Design review of the part built by this model. Coordinates are the model's own, in mm. A direction names the side the tool comes from. Coordinates: 2 decimals unless noted, no trailing zeros. Write each loop counter-clockwise with the first axis right and the second up, starting at its lowest first coordinate (ties: lowest second). Pieces come first, ordered by that corner, then holes.
Q1. Take a section at B-B (y = 12). Give the boundary of the cut face in (x, z), and give its area (3 significant figures).
Q2. Machinability: for faces 1 (the flat face through (0, 12, 12.5)), 2 (the flat face through (48, 0, 6)), 3 (the flat face through (-48, 0, -6)), which of the approach directions +Z, -Z, +X, -X, +Y, -Y give a long, thin tool a straight path to every point of the face, cutting with its end or side? Answer none if there is none.
Q3. For probe 1 along X at (y, z) = (-0.9, 0); probe 2 along Y at (x, z) = (0, 10); probe 3 along Z at (x, y) = (50, -1.3), list the stretches that pass through material, from the lowest coordinate up.
Q4. Mouldability with a two-part tool opening along X and no side actions: class faces 4 (the flat face through (-40, 0, 18)), 5 (the cylindrical face through (-45.043, -0.035, -0.651)), 6 (the flat face through (9.78, 11.13, 10.04)) as pulls with the +X half, pulls with the -X half, needs draft (parallel to the pull), parting line crosses it, or undercut.
Q5. Take a section at A-A (x = 0). Give the boundary of the cut face in (y, z), and give its area (3 significant figures).
Q6. Insertion check: pin 1 (4 mm diameter, centred on y = 0, z = 19, fed in from +X); pin 2 (4 mm diameter, centred on x = -47, y = 1, fed in from +Z); pin 3 (1.5 mm diameter, centred on x = 47, y = 1, fed in from -Z); pin 4 (8 mm diameter, centred on x = 50, z = 0, fed in from -Y). Each pin has a flat end and moves straight along its axis. Give the tip position at first contact, or say it passes through.
Q7. Take a section at D-D (z = -34). Give the boundary of the cut face in (x, y).
Q8. Take a section at C-C (y = 23.75). Give the boundary of the cut face in (x, z).
```python
from build123d import *

# Parameters (mm, degrees)
SKETCH1_R           = 5
BOSS_EXTRUDE1_DEPTH = 2.5
FILLET1_R           = 5
BOSS_EXTRUDE2_START = 10
BOSS_EXTRUDE2_DEPTH = 2.5
BOSS_EXTRUDE3_START = -10
BOSS_EXTRUDE3_DEPTH = 2.5
SKETCH3_R           = 5
CUT_EXTRUDE1_DEPTH  = 85


with BuildPart() as part:
    # Sketch1 → Boss-Extrude1 (new, symmetric)
    with BuildSketch(Plane(origin=(0, 0, 0), x_dir=(1, 0, 0), z_dir=(0, 1, 0))):
        with BuildLine():
            Line((-40, 6), (-56, 6))
            Line((-56, 6), (-56, -6))
            Line((-56, -6), (-40, -6))
            Line((-40, -6), (-40, -25))
            ThreePointArc((-40, -25), (-35.606601718, -35.606601718), (-25, -40))
            Line((-25, -40), (25, -40))
            ThreePointArc((25, -40), (35.606601718, -35.606601718), (40, -25))
            Line((40, -25), (40, -6))
            Line((40, -6), (56, -6))
            Line((56, -6), (56, 6))
            Line((56, 6), (40, 6))
            Line((40, 6), (40, 25))
            ThreePointArc((40, 25), (35.606601718, 35.606601718), (25, 40))
            Line((25, 40), (-25, 40))
            ThreePointArc((-25, 40), (-35.606601718, 35.606601718), (-40, 25))
            Line((-40, 25), (-40, 6))
        make_face()
        with Locations(Location((-50, 0, 0), (0, 0, 270))):
            Circle(SKETCH1_R, mode=Mode.SUBTRACT)
        with Locations(Location((50, 0, 0), (0, 0, 90))):
            Circle(SKETCH1_R, mode=Mode.SUBTRACT)
    extrude(amount=BOSS_EXTRUDE1_DEPTH, both=True)

    # Fillet1
    fillet1_edges = [part.edges().sort_by_distance(p)[0] for p in [
        (40, 0, -6),
        (56, 0, -6),
        (56, 0, 6),
        (40, 0, 6),
        (-40, 0, 6),
        (-56, 0, 6),
        (-56, 0, -6),
        (-40, 0, -6),
    ]]
    fillet(fillet1_edges, radius=FILLET1_R)

    # Sketch2 → Boss-Extrude2 (add, symmetric)
    with BuildSketch(Plane.XY.offset(BOSS_EXTRUDE2_START)):
        with BuildLine():
            Line((-7.5, 20), (-12, 2.5))
            Line((-12, 2.5), (12, 2.5))
            Line((12, 2.5), (7.5, 20))
            ThreePointArc((7.5, 20), (0, 27.5), (-7.5, 20))
        make_face()
    extrude(amount=BOSS_EXTRUDE2_DEPTH, both=True)

    # Sketch2_2 → Boss-Extrude3 (add, symmetric)
    with BuildSketch(Plane.XY.offset(BOSS_EXTRUDE3_START)):
        with BuildLine():
            Line((-7.5, 20), (-12, 2.5))
            Line((-12, 2.5), (12, 2.5))
            Line((12, 2.5), (7.5, 20))
            ThreePointArc((7.5, 20), (0, 27.5), (-7.5, 20))
        make_face()
    extrude(amount=BOSS_EXTRUDE3_DEPTH, both=True)

    # Sketch3 → Cut-Extrude1 (cut)
    with BuildSketch(Plane.XY.offset(12.5)):
        with Locations((0, 20)):
            Circle(SKETCH3_R)
    extrude(amount=-CUT_EXTRUDE1_DEPTH, mode=Mode.SUBTRACT)


solid = part.part
```
Response:
1. outline: (-9.56, -12.5) - (9.56, -12.5) - (9.56, -7.5) - (-9.56, -7.5) - close; (-9.56, 7.5) - (9.56, 7.5) - (9.56, 12.5) - (-9.56, 12.5) - close
1. area: 191 mm2
2. face 1: +Z, +X, -X, +Y
2. face 2: +Z, +X, +Y, -Y
2. face 3: -Z, -X, +Y, -Y
3. probe 1: x = -56 to -55, -45 to 45, 55 to 56
3. probe 2: y = -2.5 to 15, 25 to 27.5
3. probe 3: z = -6 to -5, 5 to 6
4. face 4: pulls with the -X half
4. face 5: undercut
4. face 6: pulls with the +X half
5. outline: (-2.5, -40) - (2.5, -40) - (2.5, -12.5) - (15, -12.5) - (15, -7.5) - (2.5, -7.5) - (2.5, 7.5) - (15, 7.5) - (15, 12.5) - (2.5, 12.5) - (2.5, 40) - (-2.5, 40) - close; (25, -12.5) - (27.5, -12.5) - (27.5, -7.5) - (25, -7.5) - close; (25, 7.5) - (27.5, 7.5) - (27.5, 12.5) - (25, 12.5) - close
5. area: 550 mm2
6. pin 1: stops at x = 40
6. pin 2: stops at z = 6
6. pin 3: stops at z = -6
6. pin 4: passes through
7. outline: (-37, -2.5) - (37, -2.5) - (37, 2.5) - (-37, 2.5) - close
8. outline: (-6.5, -12.5) - (-3.31, -12.5) - (-3.31, -7.5) - (-6.5, -7.5) - close; (-6.5, 7.5) - (-3.31, 7.5) - (-3.31, 12.5) - (-6.5, 12.5) - close; (3.31, -12.5) - (6.5, -12.5) - (6.5, -7.5) - (3.31, -7.5) - close; (3.31, 7.5) - (6.5, 7.5) - (6.5, 12.5) - (3.31, 12.5) - close
